Check sheet for the drawn part. Datum: minimum x, y, z corner. Units: mm. A direction names the side the tool comes from. Give positions to 0.01 mm unless a question says otherwise; leave off trailing zeros. Write each loop counter-clockwise with the first axis right and the second up, starting at its lowest first coordinate (ties: lowest second). Pieces come first, ordered by that corner, then holes. Notation, with made-up numbers: (14, 70.25) - (41, 70.25) arc R20 cw to (41, 81.25) - close; hole circle Ø6 at (-32, 34.25). An arc over 180 degrees is marked (long way). Use a Markdown table: item, result.
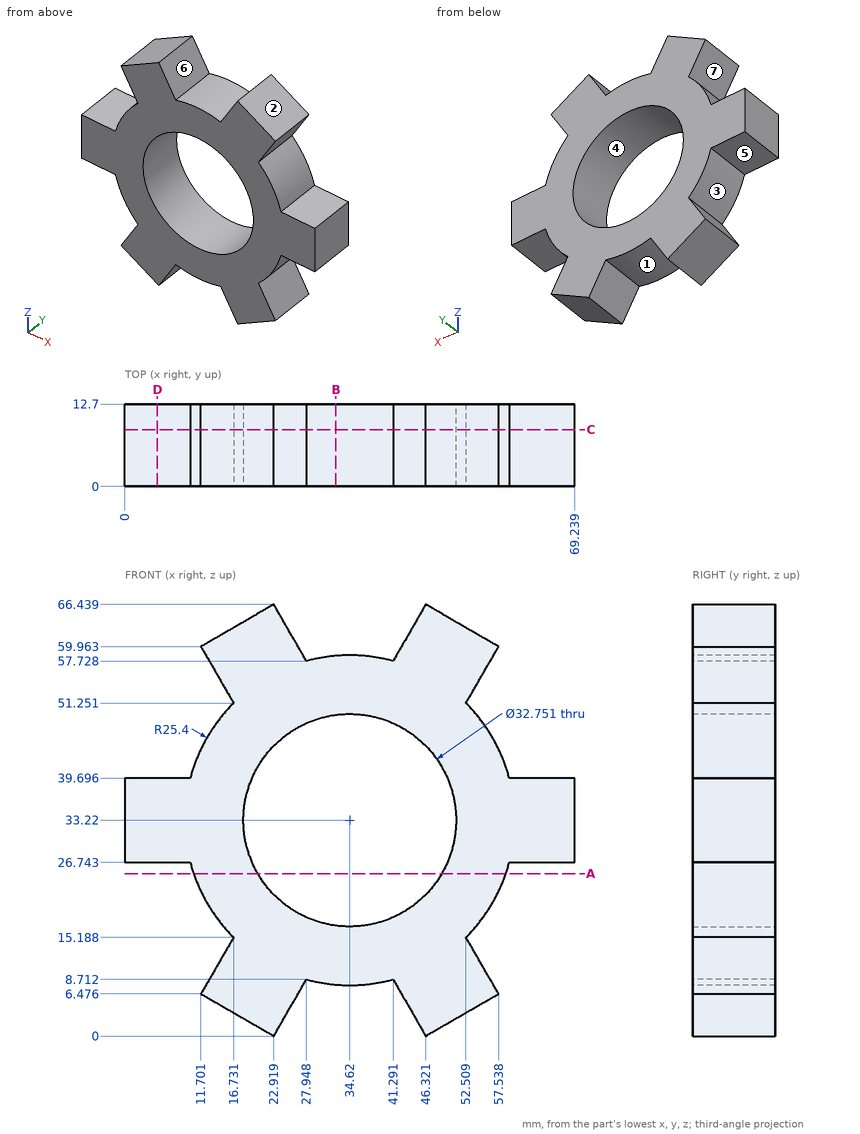
1) Section check C-C on y = 8.75. Record the boundary of the cut face in (x, z) (1 decimal), then the cut area to 3 significant figures.
Working result:
| item | result |
|---|---|
| outline | (0, 26.7) - (10.1, 26.7) arc R25.4 ccw to (16.7, 15.2) - (11.7, 6.5) - (22.9, 0) - (27.9, 8.7) arc R25.4 ccw to (41.3, 8.7) - (46.3, 0) - (57.5, 6.5) - (52.5, 15.2) arc R25.4 ccw to (59.2, 26.7) - (69.2, 26.7) - (69.2, 39.7) - (59.2, 39.7) arc R25.4 ccw to (52.5, 51.3) - (57.5, 60) - (46.3, 66.4) - (41.3, 57.7) arc R25.4 ccw to (27.9, 57.7) - (22.9, 66.4) - (11.7, 60) - (16.7, 51.3) arc R25.4 ccw to (10.1, 39.7) - (0, 39.7) - close; hole circle Ø32.8 at (34.6, 33.2) |
| area | 1,920 mm² |
2) Section check B-B on x = 32.5. Record the boundary of the cut face in (y, z).
Working result:
| item | result |
|---|---|
| outline | (0, 7.91) - (12.7, 7.91) - (12.7, 16.98) - (0, 16.98) - close; (0, 49.46) - (12.7, 49.46) - (12.7, 58.53) - (0, 58.53) - close |
3) Depth check by flat-ended pin: P1, Ø5, axis at x = 60.5, y = 3.5, coming from the -Z side (1 decimal); P2, Ø5, axis at x = 5, y = 5.5, coming from the +Z side; P3, Ø5, axis at x = 5, y = 6.5, coming from the -Z side. Enter the tip coordinate at first touch or a pass-through.
Working result:
| item | result |
|---|---|
| P1 | stops at z = 23.3 |
| P2 | stops at z = 39.7 |
| P3 | stops at z = 26.74 |
4) Set-up check for the marked faces 5, 6 and 7: record each of +Z, -Z, +X, -X, +Y, -Y from which the full face is reachable in a straight line by a thin tool's end or side.
Working result:
| item | result |
|---|---|
| face 5 | -Z, -X, +Y, -Y |
| face 6 | +Z, +Y, -Y |
| face 7 | -X, +Y, -Y |
5) Section check A-A on z = 25. Record the boundary of the cut face in (x, y).
Working result:
| item | result |
|---|---|
| outline | (10.59, 0) - (20.46, 0) - (20.46, 12.7) - (10.59, 12.7) - close; (48.78, 0) - (58.65, 0) - (58.65, 12.7) - (48.78, 12.7) - close |
6) Mould release check, pull along X, two halves, no side actions. Record for the marked faces 1, 2, 3 and 4: pulls with the +X half, pulls with the -X half, needs draft (parallel to the pull), parting line crosses it, or undercut.
Working result:
| item | result |
|---|---|
| face 1 | undercut |
| face 2 | pulls with the +X half |
| face 3 | pulls with the -X half |
| face 4 | undercut |
7) Section check D-D on x = 5. Record the boundary of the cut face in (y, z).
Working result:
| item | result |
|---|---|
| outline | (0, 26.74) - (12.7, 26.74) - (12.7, 39.7) - (0, 39.7) - close |
8) Material ranges on L1, parallel to Z at x = 35, y = 9; L2, parallel to Z at x = 63, y = 8.5; L3, parallel to X at y = 10, z = 41, recorded low to high. Write a range as from..to.
Working result:
| item | result |
|---|---|
| L1 | z = 7.82..16.85, 49.59..58.62 |
| L2 | z = 26.74..39.7 |
| L3 | x = 10.44..20.21, 49.03..58.8 |
